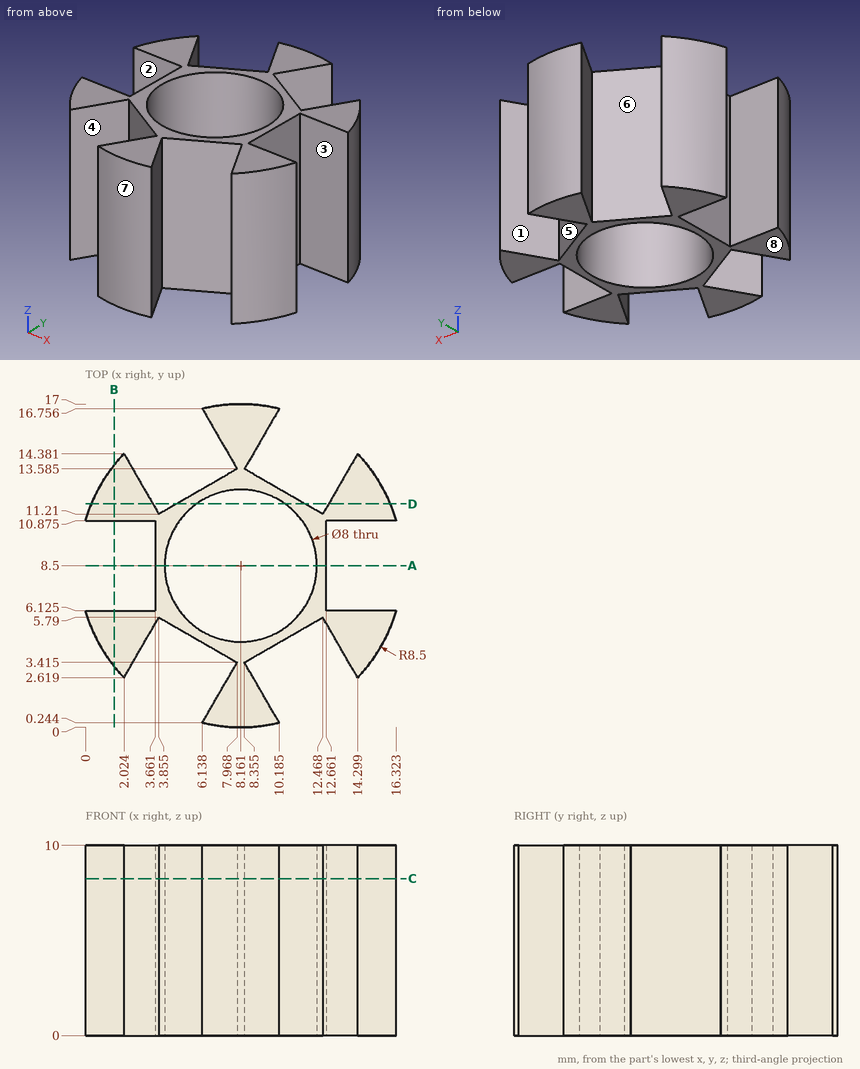
Can you work these out from the drawing? Everything is in mm from the part's minimum corner. A direction names the side the tool comes from. Coordinates: 2 decimals unless noted, no trailing zeros. Loops run counter-clockwise (first coordinate to the right, second up) from the corner with the lowest first, then second, coordinate; pieces in that order, holes last. Notation, with made-up numbers: M 30.5,57 L 35.5,57 A9 cw 35.5,61 Z; hole C 26,-14 d7. An arc over 180 degrees is marked long. Put each result on its own line as item: value. Start each with the question number.
(1) Thinking about a two-plate mould opening in Y: for the marked faces 6, 7 and 8, which applies, pulls with the +Y half, pulls with the -Y half, needs draft (parallel to the pull), parting line crosses it, or undercut?
(2) For the marked faces 1, 2, 3, 4 and 5, which set-ups out of +Z, -Z, +X, -X, +Y, -Y let a thin tool reach every point of the face, with its end or its side?
(3) Suppose I cut it at D-D on y = 11.75. Please give me the cut outline in (x, z) (1 decimal).
(4) Suppose I cut it at A-A on y = 8.5. Please give me the cut outline in (x, z).
(5) Will these pins go through, and if not, where does the flat tip stop? P1, Ø4, axis at x = 2.5, z = 3, coming from the -Y side; P2, Ø1.5, axis at y = 9.5, z = 2, coming from the -X side; P3, Ø4, axis at x = 14, z = 6.5, coming from the +Y side; P4, Ø5, axis at y = 9, z = 3.5, coming from the +X side.
(6) Suppose I cut it at C-C on z = 8.25. Please give me the cut outline in (x, y) (1 decimal).
(7) Suppose I cut it at B-B on x = 1.5. Please give me the cut outline in (y, z) (1 decimal).
(8) I need wall thicknesses on line 1 (Y direction, x = 9, z = 2.5) (1 decimal); line 2 (X direction, y = 11, z = 9.5) (1 decimal); line 3 (Y direction, x = 11, z = 5.5) (1 decimal). Which ranges of each line are inside material? Lowest first, please. Write a range as from..to.
Solutions:
1. face 6: undercut
1. face 7: pulls with the -Y half
1. face 8: needs draft
2. face 1: +Z, -Z, +Y
2. face 2: +Z, -Z, -X
2. face 3: +Z, -Z, +X
2. face 4: +Z, -Z, -Y
2. face 5: +Z, -Z
3. outline: M 0.3,0 L 3.5,0 L 3.5,10 L 0.3,10 Z; M 4.8,0 L 5.8,0 L 5.8,10 L 4.8,10 Z; M 10.5,0 L 11.5,0 L 11.5,10 L 10.5,10 Z; M 12.8,0 L 16,0 L 16,10 L 12.8,10 Z
4. outline: M 3.66,0 L 4.16,0 L 4.16,10 L 3.66,10 Z; M 12.16,0 L 12.66,0 L 12.66,10 L 12.16,10 Z
5. P1: stops at y = 2.62
5. P2: stops at x = 3.66
5. P3: stops at y = 14.38
5. P4: stops at x = 16.32
6. outline: M 0,6.1 A8.5 ccw 2,2.6 L 3.9,5.8 L 8,3.4 L 6.1,0.2 A8.5 ccw 10.2,0.2 L 8.4,3.4 L 12.5,5.8 L 14.3,2.6 A8.5 ccw 16.3,6.1 L 12.7,6.1 L 12.7,10.9 L 16.3,10.9 A8.5 ccw 14.3,14.4 L 12.5,11.2 L 8.4,13.6 L 10.2,16.8 A8.5 ccw 6.1,16.8 L 8,13.6 L 3.9,11.2 L 2,14.4 A8.5 ccw 0,10.9 L 3.7,10.9 L 3.7,6.1 Z; hole C 8.2,8.5 d8
7. outline: M 3.2,0 L 6.1,0 L 6.1,10 L 3.2,10 Z; M 10.9,0 L 13.8,0 L 13.8,10 L 10.9,10 Z
8. line 1: y = 0..2.3, 3.8..4.6, 12.4..13.2, 14.7..17
8. line 2: x = 0..5, 11.3..16.3
8. line 3: y = 4.9..5.7, 11.3..12.1
